Can you work these out from the drawing? Everything is in mm from the part's minimum corner. A direction names the side the tool comes from. Coordinates: 2 decimals unless noted, no trailing zeros. Loops run counter-clockwise (first coordinate to the right, second up) from the corner with the lowest first, then second, coordinate; pieces in that order, holes last.
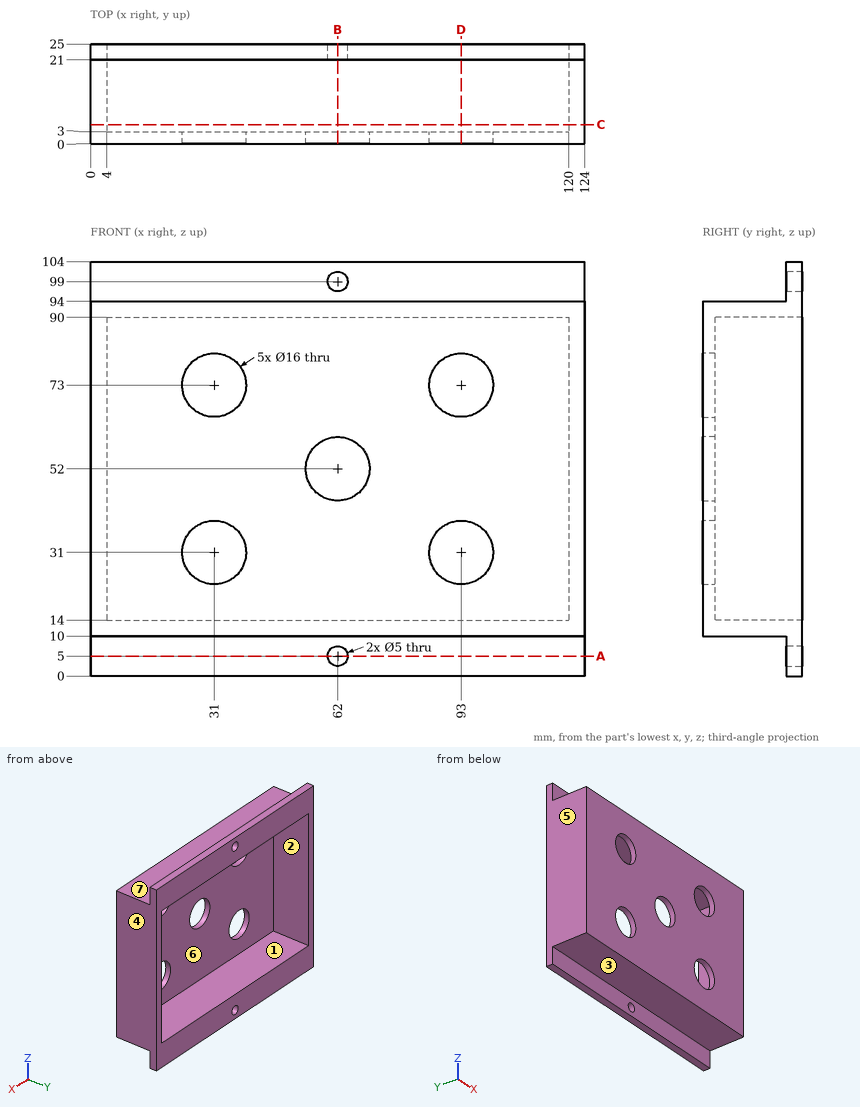
(1) Imagine slicing it at D-D, the plane x = 93. Write out the boundary of the cut face in (y, z), and give its area (3 significant figures).
Answers:
outline: (0, 10) - (21, 10) - (21, 0) - (25, 0) - (25, 14) - (3, 14) - (3, 23) - (0, 23) - close; (0, 39) - (3, 39) - (3, 65) - (0, 65) - close; (0, 81) - (3, 81) - (3, 90) - (25, 90) - (25, 104) - (21, 104) - (21, 94) - (0, 94) - close
area: 412 mm2
(2) Imagine slicing it at C-C, the plane y = 4.75. Write out the boundary of the cut face in (x, z), and give its area (3 significant figures).
Answers:
outline: (0, 10) - (124, 10) - (124, 94) - (0, 94) - close; hole (4, 14) - (120, 14) - (120, 90) - (4, 90) - close
area: 1,600 mm2
(3) Imagine slicing it at A-A, the plane z = 5. Write out the boundary of the cut face in (x, y).
Answers:
outline: (0, 21) - (59.5, 21) - (59.5, 25) - (0, 25) - close; (64.5, 21) - (124, 21) - (124, 25) - (64.5, 25) - close
(4) We'd pull the mould along X, two halves only. Please class the marked faces 1, 2, 3 and 4: +X half, -X half, draft (parallel to the pull), parting line (faces both ways), or undercut.
Answers:
face 1: undercut
face 2: undercut
face 3: draft
face 4: +X half
(5) For pin 1 (6.5 mm diameter, centred on x = 78.5, y = 13.5, fed in from -Z); pin 2 (6.5 mm diameter, centred on x = 73, y = 15, fed in from +Z); pin 3 (23 mm diameter, centred on x = 52, z = 70, fed in from +Y); pin 4 (14.5 mm diameter, centred on x = 93, z = 31, fed in from +Y), each with a flat end and sliding along its axis, tell me the tip position at first contact or that it passes through.
Answers:
pin 1: stops at z = 10
pin 2: stops at z = 94
pin 3: stops at y = 3
pin 4: passes through
(6) Imagine slicing it at B-B, the plane x = 62. Write out the boundary of the cut face in (y, z), and give its area (3 significant figures).
Answers:
outline: (0, 10) - (21, 10) - (21, 7.5) - (25, 7.5) - (25, 14) - (3, 14) - (3, 44) - (0, 44) - close; (0, 60) - (3, 60) - (3, 90) - (25, 90) - (25, 96.5) - (21, 96.5) - (21, 94) - (0, 94) - close; (21, 0) - (25, 0) - (25, 2.5) - (21, 2.5) - close; (21, 101.5) - (25, 101.5) - (25, 104) - (21, 104) - close
area: 420 mm2
(7) I need wall thicknesses on probe 1 along X at (y, z) = (2.4, 31); probe 2 along Z at (x, y) = (55, 6.5); probe 3 along X at (y, z) = (9.5, 22). Which ranges of each line are inside material? Lowest first, please.
Answers:
probe 1: x = 0 to 23, 39 to 85, 101 to 124
probe 2: z = 10 to 14, 90 to 94
probe 3: x = 0 to 4, 120 to 124
(8) Which directions (+Z, -Z, +X, -X, +Y, -Y) give clear straight access to the entire face, cutting with the end or side of a thin tool? Please do the marked faces 5, 6 and 7.
Answers:
face 5: +Z, -Z, -X, +Y, -Y
face 6: +Y
face 7: +Z, +X, -X, -Y
